```python
from build123d import *

# Parameters (mm, degrees)
F1_DEPTH = 508


# Not quite as in the source:
# - ends of sketch curves that miss each other by under 0.0002 mm in the source are joined


with BuildPart() as f1:
    # F0 (on Front) → F1 (new body)
    with BuildSketch(Plane.XZ):
        with BuildLine():
            Line((-125.4417608, 32.418528), (-110.7097608, 32.418528))
            Line((-110.7097608, 32.418528), (-110.3287608, 32.799528))
            Line((-110.3287608, 32.799528), (-109.9477608, 32.418528))
            Line((-109.9477608, 32.418528), (51.1898392, 32.418528))
            Line((51.1898392, 32.418528), (51.5708392, 32.799528))
            Line((51.5708392, 32.799528), (51.9518392, 32.418528))
            Line((51.9518392, 32.418528), (66.6838392, 32.418528))
            ThreePointArc((66.6838392, 32.418528), (70.5992308688, 34.0403363312), (72.2210392, 37.955728))
            Line((72.2210392, 37.955728), (72.2210392, 67.4102538))
            ThreePointArc((72.2210392, 67.4102538), (71.5313659528, 69.3860513433), (69.7619677468, 70.5034837164))
            ThreePointArc((69.7619677468, 70.5034837164), (69.2666914482, 70.3916273244), (69.0460392, 69.934328))
            Line((69.0460392, 69.934328), (69.0460392, 37.955728))
            ThreePointArc((69.0460392, 37.955728), (68.3541668385, 36.2854003615), (66.6838392, 35.593528))
            Line((66.6838392, 35.593528), (65.8710392, 35.593528))
            ThreePointArc((65.8710392, 35.593528), (63.6259751697, 36.5234639697), (62.6960392, 38.768528))
            Line((62.6960392, 38.768528), (62.6960392, 62.0254538))
            ThreePointArc((62.6960392, 62.0254538), (62.0063659528, 64.0012513433), (60.2369677468, 65.1186837164))
            ThreePointArc((60.2369677468, 65.1186837164), (59.7416914482, 65.0068273244), (59.5210392, 64.549528))
            Line((59.5210392, 64.549528), (59.5210392, 62.644528))
            ThreePointArc((59.5210392, 62.644528), (59.4094468836, 62.3751203164), (59.1400392, 62.263528))
            Line((59.1400392, 62.263528), (47.4052392, 62.263528))
            ThreePointArc((47.4052392, 62.263528), (46.8216542466, 61.706128041), (47.3516955482, 61.0975868915))
            Line((47.3516955482, 61.0975868915), (58.9903824, 60.0263722))
            ThreePointArc((58.9903824, 60.0263722), (59.3684465687, 59.8383423872), (59.5210392, 59.444636))
            Line((59.5210392, 59.444636), (59.5210392, 49.055528))
            ThreePointArc((59.5210392, 49.055528), (59.4094468836, 48.7861203164), (59.1400392, 48.674528))
            Line((59.1400392, 48.674528), (50.5802392, 48.674528))
            ThreePointArc((50.5802392, 48.674528), (50.1671474184, 48.5034197816), (49.9960392, 48.090328))
            Line((49.9960392, 48.090328), (49.9960392, 46.083728))
            ThreePointArc((49.9960392, 46.083728), (50.1671474184, 45.6706362184), (50.5802392, 45.499528))
            Line((50.5802392, 45.499528), (59.1400392, 45.499528))
            ThreePointArc((59.1400392, 45.499528), (59.4094468836, 45.3879356836), (59.5210392, 45.118528))
            Line((59.5210392, 45.118528), (59.5210392, 39.149528))
            ThreePointArc((59.5210392, 39.149528), (59.4094468836, 38.8801203164), (59.1400392, 38.768528))
            Line((59.1400392, 38.768528), (50.3770392, 38.768528))
            ThreePointArc((50.3770392, 38.768528), (50.1076315164, 38.6569356836), (49.9960392, 38.387528))
            Line((49.9960392, 38.387528), (49.9960392, 35.974528))
            ThreePointArc((49.9960392, 35.974528), (49.8844468836, 35.7051203164), (49.6150392, 35.593528))
            Line((49.6150392, 35.593528), (-29.1249608, 35.593528))
            Line((-29.1249608, 35.593528), (-29.3789608, 35.339528))
            Line((-29.3789608, 35.339528), (-29.6329608, 35.593528))
            Line((-29.6329608, 35.593528), (-108.3729608, 35.593528))
            ThreePointArc((-108.3729608, 35.593528), (-108.6423684836, 35.7051203164), (-108.7539608, 35.974528))
            Line((-108.7539608, 35.974528), (-108.7539608, 38.387528))
            ThreePointArc((-108.7539608, 38.387528), (-108.8655531164, 38.6569356836), (-109.1349608, 38.768528))
            Line((-109.1349608, 38.768528), (-117.8979608, 38.768528))
            ThreePointArc((-117.8979608, 38.768528), (-118.1673684836, 38.8801203164), (-118.2789608, 39.149528))
            Line((-118.2789608, 39.149528), (-118.2789608, 45.118528))
            ThreePointArc((-118.2789608, 45.118528), (-118.1673684836, 45.3879356836), (-117.8979608, 45.499528))
            Line((-117.8979608, 45.499528), (-109.3381608, 45.499528))
            ThreePointArc((-109.3381608, 45.499528), (-108.9250690184, 45.6706362184), (-108.7539608, 46.083728))
            Line((-108.7539608, 46.083728), (-108.7539608, 48.090328))
            ThreePointArc((-108.7539608, 48.090328), (-108.9250690184, 48.5034197816), (-109.3381608, 48.674528))
            Line((-109.3381608, 48.674528), (-117.8979608, 48.674528))
            ThreePointArc((-117.8979608, 48.674528), (-118.1673684836, 48.7861203164), (-118.2789608, 49.055528))
            Line((-118.2789608, 49.055528), (-118.2789608, 59.444636))
            ThreePointArc((-118.2789608, 59.444636), (-118.1263681687, 59.8383423872), (-117.7483044518, 60.0263771085))
            Line((-117.7483044518, 60.0263771085), (-106.1096176, 61.0975918))
            ThreePointArc((-106.1096176, 61.0975918), (-105.5795758466, 61.706128041), (-106.1631608, 62.263528))
            Line((-106.1631608, 62.263528), (-117.4788608, 62.263528))
            ThreePointArc((-117.4788608, 62.263528), (-118.0446169356, 62.4978718644), (-118.2789608, 63.063628))
            ThreePointArc((-118.2789608, 63.063628), (-118.0446169356, 63.6293841356), (-117.4788608, 63.863728))
            Line((-117.4788608, 63.863728), (-114.1387608, 63.863728))
            ThreePointArc((-114.1387608, 63.863728), (-113.6897479939, 64.0497151939), (-113.5037608, 64.498728))
            ThreePointArc((-113.5037608, 64.498728), (-113.6897479939, 64.9477408061), (-114.1387608, 65.133728))
            Line((-114.1387608, 65.133728), (-118.2789608, 65.133728))
            ThreePointArc((-118.2789608, 65.133728), (-120.5240248303, 64.2037920303), (-121.4539608, 61.958728))
            Line((-121.4539608, 61.958728), (-121.4539608, 38.768528))
            ThreePointArc((-121.4539608, 38.768528), (-122.3838967697, 36.5234639697), (-124.6289608, 35.593528))
            Line((-124.6289608, 35.593528), (-125.4417608, 35.593528))
            ThreePointArc((-125.4417608, 35.593528), (-127.1120884385, 36.2854003615), (-127.8039608, 37.955728))
            Line((-127.8039608, 37.955728), (-127.8039608, 69.934328))
            ThreePointArc((-127.8039608, 69.934328), (-128.0246130482, 70.3916273244), (-128.5198891538, 70.503482883))
            ThreePointArc((-128.5198891538, 70.503482883), (-130.2892875528, 69.3860513433), (-130.9789608, 67.4102538))
            Line((-130.9789608, 67.4102538), (-130.9789608, 37.955728))
            ThreePointArc((-130.9789608, 37.955728), (-129.3571524688, 34.0403363312), (-125.4417608, 32.418528))
        make_face()
    extrude(amount=F1_DEPTH)


solid = f1.part
```
Here's how the part is built. I have some questions about the finished solid (model axes, mm). A direction names the side the tool comes from. Coordinates: 2 decimals unless noted, no trailing zeros. Loops run counter-clockwise (first coordinate to the right, second up) from the corner with the lowest first, then second, coordinate; pieces in that order, holes last. Notation, with made-up numbers: M 20,54.25 L 55,54.25 A32 cw 55,82.25 Z; hole C 83,9.5 d2. An arc over 180 degrees is marked long. One line per item, written item: value.
1. Thinking about a two-plate mould opening in Z: for faces 4 (the flat face through (59, -250, 32.419)), 5 (the flat face through (-127.804, -250, 54)), 6 (the flat face through (59.521, -250, 54)), which applies, +Z half, -Z half, draft (parallel to the pull), parting line (faces both ways), or undercut?
Geometry says:
face 4: -Z half
face 5: draft
face 6: undercut
2. Imagine slicing it at A-A (z = 54). List the corners of the cut face in (x, y) for me, and give its area (3 significant figures).
Geometry says:
outline: M -130.98,-508 L -127.8,-508 L -127.8,0 L -130.98,0 Z; M -121.45,-508 L -118.28,-508 L -118.28,0 L -121.45,0 Z; M 59.52,-508 L 62.7,-508 L 62.7,0 L 59.52,0 Z; M 69.05,-508 L 72.22,-508 L 72.22,0 L 69.05,0 Z
area: 6,450 mm2
3. Will these pins go through, and if not, where does the flat tip stop? pin 1 Ø4.5 at (x, y) = (56, -380) entering from +Z; pin 2 Ø9.5 at (x, y) = (-112, -303.5) entering from +Z; pin 3 Ø10 at (x, z) = (-70, 43) entering from -Y; pin 4 Ø0.7 at (x, y) = (-125, -139) entering from +Z.
Geometry says:
pin 1: stops at z = 62.26
pin 2: stops at z = 65.13
pin 3: passes through
pin 4: stops at z = 35.59
4. Imagine slicing it at B-B (x = -45). List the corners of the cut face in (y, z) for me.
Geometry says:
outline: M -508,32.42 L 0,32.42 L 0,35.59 L -508,35.59 Z
5. On a 3-axis mill with a long thin cutter (end or side, diameter ignored), from which of +Z, -Z, +X, -X, +Y, -Y can I reach the whole of each face in a straight line? I mean faces 1 (the flat face through (-118, -250, 32.419)), 2 (the flat face through (55, -250, 45.5)), 3 (the flat face through (-121.454, -250, 51)). Say none if no direction works.
Geometry says:
face 1: -Z, +X, -X, +Y, -Y
face 2: +Y, -Y
face 3: +Z, +Y, -Y
6. Please list where these lines run through material, in increasing order: probe 1 along X at (y, z) = (-240.5, 48); probe 2 along X at (y, z) = (-413, 43); probe 3 along Z at (x, y) = (-117.5, -171.5).
Geometry says:
probe 1: x = -130.98 to -127.8, -121.45 to -108.75, 50 to 62.7, 69.05 to 72.22
probe 2: x = -130.98 to -127.8, -121.45 to -118.28, 59.52 to 62.7, 69.05 to 72.22
probe 3: z = 32.42 to 38.77, 45.5 to 48.67, 60.05 to 62.26, 63.86 to 65.13
